```python
from build123d import *

# Parameters (mm, degrees)
F0_R     = 7.35
F1_DEPTH = 16.5
F2_R     = 4.45
F3_DEPTH = 7.08
F6_DEPTH = 4.83
F7_R     = 2.25
F8_DEPTH = 25
F9_DEPTH = 25


with BuildPart() as f1:
    # F0 (on Top) → F1 (new body)
    with BuildSketch(Plane.XY):
        Circle(F0_R)
    extrude(amount=F1_DEPTH)

    # F2 (on face) → F3 (join)
    with BuildSketch(Plane.XY.offset(16.5)):
        Circle(F2_R)
    extrude(amount=F3_DEPTH)

    # F5 (on face) → F6 (join)
    with BuildSketch(Plane.XY.offset(23.58)):
        with BuildLine():
            Line((0, -1.75), (0, 1.75))
            ThreePointArc((0, 1.75), (-1.75, 0), (0, -1.75))
        make_face()
    extrude(amount=F6_DEPTH)

    # F7 (on face) → F8 (cut)
    with BuildSketch(Plane(origin=(0, 0, 0), x_dir=(1, 0, 0), z_dir=(0, 0, -1))):
        with Locations((0, -9)):
            Circle(F7_R)
        with Locations((5.2900672706, -7.2811529494)):
            Circle(F7_R)
        with Locations((8.5595086467, -2.7811529494)):
            Circle(F7_R)
        with Locations((8.5595086467, 2.7811529494)):
            Circle(F7_R)
        with Locations((5.2900672706, 7.2811529494)):
            Circle(F7_R)
        with Locations((0, 9)):
            Circle(F7_R)
        with Locations((-5.2900672706, 7.2811529494)):
            Circle(F7_R)
        with Locations((-8.5595086467, 2.7811529494)):
            Circle(F7_R)
        with Locations((-8.5595086467, -2.7811529494)):
            Circle(F7_R)
        with Locations((-5.2900672706, -7.2811529494)):
            Circle(F7_R)
    extrude(amount=-F8_DEPTH, mode=Mode.SUBTRACT)

    # F7 (on face) → F9 (cut)
    with BuildSketch(Plane(origin=(0, 0, 0), x_dir=(1, 0, 0), z_dir=(0, 0, -1))):
        with BuildLine():
            ThreePointArc((7.2919167208, -0.9221987516), (6.419631485, -2.085864712), (6.4413393745, -3.5400066472))
            ThreePointArc((6.4413393745, -3.5400066472), (6.9902653948, -2.2712749087), (7.2919167208, -0.9221987516))
        make_face()
        with BuildLine():
            ThreePointArc((5.3572297228, -5.0321555716), (4.3202216043, -5.9462749087), (3.1303893203, -6.6500498271))
            ThreePointArc((3.1303893203, -6.6500498271), (4.9713004187, -9.5084579788), (7.5400672706, -7.2811529494))
            ThreePointArc((7.5400672706, -7.2811529494), (6.9046284366, -5.7140881003), (5.3572297228, -5.0321555716))
        make_face()
        with BuildLine():
            ThreePointArc((-1.3762630563, -7.22), (-0.9914403975, -11.0197885875), (2.25, -9))
            ThreePointArc((2.25, -9), (2.0197885875, -8.0085596025), (1.3762630563, -7.22))
            ThreePointArc((1.3762630563, -7.22), (0, -7.35), (-1.3762630563, -7.22))
        make_face()
        with BuildLine():
            ThreePointArc((-3.0400672706, -7.2811529494), (-3.0627622412, -6.9623860974), (-3.1303893203, -6.6500498271))
            ThreePointArc((-3.1303893203, -6.6500498271), (-4.3202216043, -5.9462749087), (-5.3572297228, -5.0321555716))
            ThreePointArc((-5.3572297228, -5.0321555716), (-6.8571321197, -8.8957141153), (-3.0400672706, -7.2811529494))
        make_face()
        with BuildLine():
            ThreePointArc((-7.2919167208, -0.9221987516), (-10.6993858083, -3.4764411867), (-6.4413393745, -3.5400066472))
            ThreePointArc((-6.4413393745, -3.5400066472), (-6.9902653948, -2.2712749087), (-7.2919167208, -0.9221987516))
        make_face()
        with BuildLine():
            ThreePointArc((-6.4413393745, 3.5400066472), (-10.6993858083, 3.4764411867), (-7.2919167208, 0.9221987516))
            ThreePointArc((-7.2919167208, 0.9221987516), (-6.9902653948, 2.2712749087), (-6.4413393745, 3.5400066472))
        make_face()
        with BuildLine():
            ThreePointArc((-3.1303893203, 6.6500498271), (-4.3202216043, 5.9462749087), (-5.3572297228, 5.0321555716))
            ThreePointArc((-5.3572297228, 5.0321555716), (-3.967550453, 5.460864712), (-3.1303893203, 6.6500498271))
        make_face()
        with BuildLine():
            ThreePointArc((1.3762630563, 7.22), (0, 7.35), (-1.3762630563, 7.22))
            ThreePointArc((-1.3762630563, 7.22), (0, 6.75), (1.3762630563, 7.22))
        make_face()
        with BuildLine():
            ThreePointArc((3.1303893203, 6.6500498271), (3.967550453, 5.460864712), (5.3572297228, 5.0321555716))
            ThreePointArc((5.3572297228, 5.0321555716), (4.3202216043, 5.9462749087), (3.1303893203, 6.6500498271))
        make_face()
        with BuildLine():
            ThreePointArc((6.4413393745, 3.5400066472), (6.419631485, 2.085864712), (7.2919167208, 0.9221987516))
            ThreePointArc((7.2919167208, 0.9221987516), (6.9902653948, 2.2712749087), (6.4413393745, 3.5400066472))
        make_face()
    extrude(amount=-F9_DEPTH, mode=Mode.SUBTRACT)


solid = f1.part
```
CAD build for the part. Positions are in the model's coordinates, mm. A direction names the side the tool comes from. Round coordinates to 2 decimals unless told otherwise and drop trailing zeros. Order: outer loops, then holes, each group sorted by start corner. A loop starts at its lowest first (then second) coordinate and runs counter-clockwise, first axis right, second up. Notation, with made-up numbers: (-16, -34) -> (34, -34) arc R26 ccw to (34, -17) -> close; hole circle Ø4 at (-31.75, 55.5). An arc over 180 degrees is marked (long way). Write item = value, one per line.
(1) 3-axis set-ups, long thin cutter, end or side, ignore diameter. For faces 4 (the cylindrical face through (2.259, -6.994, 8.134)), 5 (the cylindrical face through (-2.259, 6.994, 8.134)), 6 (the cylindrical face through (-0.965, -4.344, 19.99)), 7 (the cylindrical face through (-1.75, 0.04, 25.96)), 8 (the flat face through (0, 0, 26)): which of +Z, -Z, +X, -X, +Y, -Y reach the whole face in a straight line?
Answers follow:
face_4 = +Z, -Z, +X, -Y
face_5 = +Z, -Z, -X, +Y
face_6 = +Z
face_7 = +Z, -X
face_8 = +Z, +X, +Y, -Y
(2) Cut at D-D (x = 1). Write the cut outline in (y, z).
Answers follow:
outline = (-6.98, 0) -> (6.98, 0) -> (6.98, 16.5) -> (4.34, 16.5) -> (4.34, 23.58) -> (-4.34, 23.58) -> (-4.34, 16.5) -> (-6.98, 16.5) -> close
(3) Cut at B-B (z = 15.25). Write the cut outline in (x, y), plus the area to 3 significant figures.
Answers follow:
outline = (-7.29, -0.92) arc R2.25 cw to (-6.44, -3.54) arc R7.35 ccw to (-5.36, -5.03) arc R2.25 cw to (-3.13, -6.65) arc R7.35 ccw to (-1.38, -7.22) arc R2.25 cw to (1.38, -7.22) arc R7.35 ccw to (3.13, -6.65) arc R2.25 cw to (5.36, -5.03) arc R7.35 ccw to (6.44, -3.54) arc R2.25 cw to (7.29, -0.92) arc R7.35 ccw to (7.29, 0.92) arc R2.25 cw to (6.44, 3.54) arc R7.35 ccw to (5.36, 5.03) arc R2.25 cw to (3.13, 6.65) arc R7.35 ccw to (1.38, 7.22) arc R2.25 cw to (-1.38, 7.22) arc R7.35 ccw to (-3.13, 6.65) arc R2.25 cw to (-5.36, 5.03) arc R7.35 ccw to (-6.44, 3.54) arc R2.25 cw to (-7.29, 0.92) arc R7.35 ccw to start
area = 159 mm²
(4) Drill centre lines: L1, parallel to Z at x = 6.5, y = 0.5; L2, parallel to Z at x = -2.75, y = -0.5; L3, parallel to X at y = 2.75, z = 12.75. Where is each one in solid material? Low to high.
Answers follow:
L1 = 0 to 16.5
L2 = 0 to 23.58
L3 = -6.31 to 6.31
(5) Flat gauge pins, fed straight in: P1, Ø3, axis at y = -4, z = 9.5, coming from the +X side; P2, Ø8, axis at x = -6, z = 14, coming from the -Y side; P3, Ø8, axis at y = 5.5, z = 15, coming from the -X side. Where does each tip first touch, or does it go through?
Answers follow:
P1 = 6.44
P2 = -7.07
P3 = -6.71
(6) Cut at C-C (x = -3.75). Write the cut outline in (y, z), plus the area to 3 significant figures.
Answers follow:
outline = (-5.64, 0) -> (5.64, 0) -> (5.64, 16.5) -> (2.4, 16.5) -> (2.4, 23.58) -> (-2.4, 23.58) -> (-2.4, 16.5) -> (-5.64, 16.5) -> close
area = 220 mm²
(7) Pull direction Y, two halves, no side cores. Call faces 1 (the cylindrical face through (3.98, 5.45, 8.13)), 2 (the cylindrical face through (7.35, -0.01, 8.13)), 3 (the cylindrical face through (6.41, -2.11, 8.13)): +Y half, -Y half, draft (parallel to the pull), parting line (faces both ways), or undercut.
Answers follow:
face_1 = +Y half
face_2 = parting line
face_3 = undercut
(8) Cut at A-A (y = 0). Write the cut outline in (x, z).
Answers follow:
outline = (-7.35, 0) -> (7.35, 0) -> (7.35, 16.5) -> (4.45, 16.5) -> (4.45, 23.58) -> (0, 23.58) -> (0, 28.41) -> (-1.75, 28.41) -> (-1.75, 23.58) -> (-4.45, 23.58) -> (-4.45, 16.5) -> (-7.35, 16.5) -> close
